Can you work these out from the model? Positions are in its coordinate system, mm. A direction names the side the tool comes from. Round coordinates to 2 decimals unless told otherwise and drop trailing zeros. Loops run counter-clockwise (first coordinate to the right, second up) from the corner with the lowest first, then second, coordinate; pieces in that order, holes last. Notation, with made-up numbers: (69, -26) -> (121, -26) arc R9 ccw to (121, -19) -> close; hole circle Ø7 at (53.5, 80). An arc over 180 degrees is marked (long way). Use a Markdown table: item, result.
from build123d import *

# Parameters (mm, degrees)
SKETCH1_W               = 26
SKETCH1_H               = 41
SKETCH1_R               = 1.375
SKETCH1_R_2             = 0.925
SKETCH1_H_2             = 4.4
BOSS_EXTRUDE1_DEPTH     = 6
SKETCH2_R               = 0.925
SKETCH2_R_2             = 1.375
BOSS_EXTRUDE2_DEPTH     = 15
CUT_EXTRUDE2_DEPTH      = 42.677451937
CUT_EXTRUDE2_DEPTH_BACK = 42.677451937
SKETCH4_W               = 26
SKETCH4_H               = 45.4
CUT_EXTRUDE1_DEPTH      = 7
FILLET1_R               = 2.2
FILLET2_R               = 2.2


with BuildPart() as part:
    # Sketch1 → Boss-Extrude1 (new body)
    # profile 1 of 2: a face of its own
    with BuildSketch(Plane(origin=(0, 0, 0), x_dir=(1, 0, 0), z_dir=(0, 1, 0))):
        Rectangle(SKETCH1_W, SKETCH1_H)
        with Locations(Location((-9, -18, 0), (0, 0, 270))):
            Circle(SKETCH1_R, mode=Mode.SUBTRACT)
        with BuildLine():
            ThreePointArc((10.375, -18), (9, -19.375), (7.625, -18))
            ThreePointArc((7.625, -18), (9, -16.625), (10.375, -18))
        make_face(mode=Mode.SUBTRACT)
        with Locations(Location((-9.5, 16, 0), (0, 0, 270))):
            Circle(SKETCH1_R_2, mode=Mode.SUBTRACT)
        with BuildLine():
            ThreePointArc((10.425, 16), (9.5, 15.075), (8.575, 16))
            ThreePointArc((8.575, 16), (9.5, 16.925), (10.425, 16))
        make_face(mode=Mode.SUBTRACT)
    # profile 2 of 2: a face of its own
    with BuildSketch(Plane(origin=(0, 0, 0), x_dir=(1, 0, 0), z_dir=(0, 1, 0))):
        with Locations((0, -22.7)):
            Rectangle(SKETCH1_W, SKETCH1_H_2)
    extrude(amount=BOSS_EXTRUDE1_DEPTH)

    # Sketch2 → Boss-Extrude2 (add)
    # profile 1 of 6: a face of its own
    with BuildSketch(Plane(origin=(0, 6, 0), x_dir=(1, 0, 0), z_dir=(0, 1, 0))):
        Polygon((12.587244228, 16.385905528), (10.85066935, 17.736574878), (9.114094472, 19.087244228), (0, 2.5), (4, 2.5), (4, 0), align=None)
        with BuildLine():
            ThreePointArc((10.425, 16), (8.669058384, 15.593599912), (10.067895068, 16.730150801))
            ThreePointArc((10.067895068, 16.730150801), (10.330941616, 16.406400088), (10.425, 16))
        make_face(mode=Mode.SUBTRACT)
    # profile 2 of 6: a face of its own
    with BuildSketch(Plane(origin=(0, 6, 0), x_dir=(1, 0, 0), z_dir=(0, 1, 0))):
        Polygon((-4, 0), (-4, 2.5), (0, 2.5), (-9.114094472, 19.087244228), (-12.587244228, 16.385905528), align=None)
        with Locations(Location((-9.5, 16, 0), (0, 0, 270))):
            Circle(SKETCH2_R, mode=Mode.SUBTRACT)
    # profile 3 of 6: a face of its own
    with BuildSketch(Plane(origin=(0, 6, 0), x_dir=(1, 0, 0), z_dir=(0, 1, 0))):
        Polygon((0, 2.5), (-4, 2.5), (-4, 0), (-4, -2.5), (0, -2.5), align=None)
    # profile 4 of 6: a face of its own
    with BuildSketch(Plane(origin=(0, 6, 0), x_dir=(1, 0, 0), z_dir=(0, 1, 0))):
        Polygon((4, 2.5), (0, 2.5), (0, -2.5), (4, -2.5), (4, 0), align=None)
    # profile 5 of 6: a face of its own
    with BuildSketch(Plane(origin=(0, 6, 0), x_dir=(1, 0, 0), z_dir=(0, 1, 0))):
        Polygon((12.482501962, -18.524099305), (4, 0), (4, -2.5), (0, -2.5), (7.724231954, -21.282516701), (10.103366958, -19.903308003), align=None)
        with BuildLine():
            ThreePointArc((10.375, -18), (10.191392249, -18.686447019), (9.689604349, -19.189567502))
            ThreePointArc((9.689604349, -19.189567502), (7.808607751, -17.313552981), (10.375, -18))
        make_face(mode=Mode.SUBTRACT)
    # profile 6 of 6: a face of its own
    with BuildSketch(Plane(origin=(0, 6, 0), x_dir=(1, 0, 0), z_dir=(0, 1, 0))):
        Polygon((-4, -2.5), (-4, 0), (-12.482501962, -18.524099305), (-7.724231954, -21.282516701), (0, -2.5), align=None)
        with Locations(Location((-9, -18, 0), (0, 0, 270))):
            Circle(SKETCH2_R_2, mode=Mode.SUBTRACT)
    extrude(amount=BOSS_EXTRUDE2_DEPTH)

    # Sketch6 → Cut-Extrude2 (cut, two sides: drawn at the far end of the back side and taken through both)
    with BuildSketch(Plane(origin=(13, 0, 0), x_dir=(0, 0, -1), z_dir=(1, 0, 0)).offset(-CUT_EXTRUDE2_DEPTH_BACK)):
        Polygon((-21.28, 17), (-21.28, 11), (-12.8, 11), (10.59, 17), align=None)
        Polygon((10.59, 12), (-12.8, 6), (19.09, 6), (19.09, 12), align=None)
        Polygon((-21.28, 21.511868699), (-21.28, 17), (10.59, 17), (19.087244228, 17), (19.087244228, 21.511868699), align=None)
    extrude(amount=CUT_EXTRUDE2_DEPTH + CUT_EXTRUDE2_DEPTH_BACK, mode=Mode.SUBTRACT)

    # Sketch4 → Cut-Extrude1 (cut)
    with BuildSketch(Plane.XZ):
        with Locations((0, 2.2)):
            Rectangle(SKETCH4_W, SKETCH4_H)
    extrude(amount=-CUT_EXTRUDE1_DEPTH, mode=Mode.SUBTRACT)

    # Fillet1
    # the kernel refuses this fillet: 2.2 mm, written as the material it takes off along each edge
    with BuildSketch(Plane(origin=(12.587244228, 7.402722975, -16.385905528), x_dir=(-0.46418305146339667, 0, 0.8857392927572592), z_dir=(0, 1, 0))) as fillet1_piece_1:
        with BuildLine():
            CenterArc((FILLET1_R * 0.83586855008, -FILLET1_R), FILLET1_R, 90, 79.782379698)
            Line((-FILLET1_R * 0.148272552074, -FILLET1_R * 0.822612596131), (0, 0))
            Line((0, 0), (FILLET1_R * 0.83586855008, 0))
        make_face()
    extrude(amount=14.194554051, mode=Mode.SUBTRACT)
    with BuildSketch(Plane(origin=(9.114094472, 5.550330565, -19.087244228), x_dir=(-0.48155808709989106, 0, 0.8764141764877459), z_dir=(0, 1, 0))) as fillet1_piece_2:
        with BuildLine():
            CenterArc((FILLET1_R * 1.17266716994, FILLET1_R), FILLET1_R, 170.912229019, 99.087770981)
            Line((FILLET1_R * 0.185219628956, FILLET1_R * 1.15794731336), (0, 0))
            Line((0, 0), (FILLET1_R * 1.17266716994, 0))
        make_face()
    extrude(amount=17.899338869, mode=Mode.SUBTRACT)
    with BuildSketch(Plane(origin=(-9.114094472, 5.550330565, -19.087244228), x_dir=(0.4815580870998917, 0, 0.8764141764877456), z_dir=(0, 1, 0))) as fillet1_piece_3:
        with BuildLine():
            CenterArc((FILLET1_R * 1.17266716994, -FILLET1_R), FILLET1_R, 90, 99.087770981)
            Line((FILLET1_R * 0.185219628956, -FILLET1_R * 1.15794731336), (0, 0))
            Line((0, 0), (FILLET1_R * 1.17266716994, 0))
        make_face()
    extrude(amount=17.899338869, mode=Mode.SUBTRACT)
    with BuildSketch(Plane(origin=(-12.587244228, 7.402722975, -16.385905528), x_dir=(0.46418305146339667, 0, 0.8857392927572592), z_dir=(0, 1, 0))) as fillet1_piece_4:
        with BuildLine():
            CenterArc((FILLET1_R * 0.83586855008, FILLET1_R), FILLET1_R, 190.217620302, 79.782379698)
            Line((-FILLET1_R * 0.148272552074, FILLET1_R * 0.822612596131), (0, 0))
            Line((0, 0), (FILLET1_R * 0.83586855008, 0))
        make_face()
    extrude(amount=14.194554051, mode=Mode.SUBTRACT)
    with BuildSketch(Plane(origin=(-12.482501962, 2.003928442, 18.524099305), x_dir=(0.4163419464168799, 0, -0.9092081080004752), z_dir=(0, 1, 0))) as fillet1_piece_5:
        with BuildLine():
            CenterArc((FILLET1_R * 0.908376646875, -FILLET1_R), FILLET1_R, 90, 84.502549141)
            Line((-FILLET1_R * 0.087023814771, -FILLET1_R * 0.904198533648), (0, 0))
            Line((0, 0), (FILLET1_R * 0.908376646875, 0))
        make_face()
    extrude(amount=13.992143116, mode=Mode.SUBTRACT)
    with BuildSketch(Plane(origin=(-7.724231954, 0.701160202, 21.282516701), x_dir=(0.3803394674675552, 0, -0.9248469546289788), z_dir=(0, 1, 0))) as fillet1_piece_6:
        with BuildLine():
            CenterArc((FILLET1_R * 1.14524359963, FILLET1_R), FILLET1_R, 172.25340707, 97.74659293)
            Line((FILLET1_R * 0.154369685137, FILLET1_R * 1.13479200861), (0, 0))
            Line((0, 0), (FILLET1_R * 1.14524359963, 0))
        make_face()
    extrude(amount=26.597679596, mode=Mode.SUBTRACT)
    with BuildSketch(Plane(origin=(12.482501962, 2.003928442, 18.524099305), x_dir=(-0.4163419464168806, 0, -0.9092081080004749), z_dir=(0, 1, 0))) as fillet1_piece_7:
        with BuildLine():
            CenterArc((FILLET1_R * 0.908376646875, FILLET1_R), FILLET1_R, 185.497450859, 84.502549141)
            Line((-FILLET1_R * 0.087023814771, FILLET1_R * 0.904198533648), (0, 0))
            Line((0, 0), (FILLET1_R * 0.908376646875, 0))
        make_face()
    extrude(amount=13.992143116, mode=Mode.SUBTRACT)
    with BuildSketch(Plane(origin=(7.724231954, 0.701160202, 21.282516701), x_dir=(-0.38033946746755576, 0, -0.9248469546289787), z_dir=(0, 1, 0))) as fillet1_piece_8:
        with BuildLine():
            CenterArc((FILLET1_R * 1.14524359963, -FILLET1_R), FILLET1_R, 90, 97.74659293)
            Line((FILLET1_R * 0.154369685137, -FILLET1_R * 1.13479200861), (0, 0))
            Line((0, 0), (FILLET1_R * 1.14524359963, 0))
        make_face()
    extrude(amount=26.597679596, mode=Mode.SUBTRACT)

    # Fillet2
    fillet2_edges = [part.edges().sort_by_distance(p)[0] for p in [
        (-4, 11.783454468, 0),
        (0, 12.424754168, -2.5),
        (4, 11.783454468, 0),
        (0, 11.142154767, 2.5),
    ]]
    fillet(fillet2_edges, radius=FILLET2_R)


solid = part.part
1. I need wall thicknesses on line 1 (X direction, y = 8.95, z = 18) (3 decimals); line 2 (X direction, y = 15.75, z = -15.5); line 3 (Y direction, x = 6.75, z = 17.5). Which ranges of each line are inside material? Lowest first, please.
Answer sheet:
| item | result |
|---|---|
| line 1 | x = -11.818 to -10.375, -7.625 to -6.374, 6.374 to 7.625, 10.375 to 11.818 |
| line 2 | x = -11.97 to -10.28, -8.72 to -7.14, 7.14 to 8.72, 10.28 to 11.97 |
| line 3 | y = 7 to 11 |
2. Will these pins go through, and if not, where does the flat tip stop? pin 1 Ø1.7 at (x, z) = (9, 18) entering from +Y; pin 2 Ø6 at (x, z) = (9.5, 16) entering from +Y; pin 3 Ø2 at (x, z) = (8, -15.5) entering from -Y; pin 4 Ø5 at (y, z) = (10, 6) entering from -X.
Answer sheet:
| item | result |
|---|---|
| pin 1 | passes through |
| pin 2 | stops at y = 11 |
| pin 3 | stops at y = 12 |
| pin 4 | stops at x = -7.89 |
3. I want a section at A-A (x = -5.25). Please give me the cut outline in (y, z).
Answer sheet:
| item | result |
|---|---|
| outline | (7, 8.9) -> (8.58, 2.73) -> (13.58, 2.73) -> (11, 12.8) -> (11, 15.27) -> (7, 15.27) -> close; (9.9, -2.39) -> (12, -10.59) -> (12, -12.05) -> (17, -12.05) -> (17, -10.59) -> (14.9, -2.39) -> close |
4. I want a section at D-D (x = 6). Please give me the cut outline in (y, z), plus the area to 3 significant figures.
Answer sheet:
| item | result |
|---|---|
| outline | (7, 8.9) -> (8.16, 4.37) -> (13.16, 4.37) -> (11, 12.8) -> (11, 17.09) -> (7, 17.09) -> close; (10.26, -3.82) -> (12, -10.59) -> (12, -13.42) -> (17, -13.42) -> (17, -10.59) -> (15.26, -3.82) -> close |
| area | 105 mm² |
5. If we mould it in two halves opening along Z, with no side actions, what happens to faces 1 (the cylindrical face through (-8.87, 14.46, -16.68)), 2 (the cylindrical face through (-8.1, 9, 20.2)), 3 (the flat face through (-8, 12, -14))? For each: +Z half, -Z half, draft (parallel to the pull), parting line (faces both ways), or undercut.
Answer sheet:
| item | result |
|---|---|
| face 1 | undercut |
| face 2 | +Z half |
| face 3 | draft |
6. Which directions (+Z, -Z, +X, -X, +Y, -Y) give clear straight access to the entire face, cutting with the end or side of a thin tool? Please do faces 4 (the flat face through (-8, 11, 16)), 5 (the flat face through (-8.168, 14.042, -7.953)), 6 (the flat face through (8.067, 14.042, -7.76)), 7 (the flat face through (4.94, 14.56, -11.49)).
Answer sheet:
| item | result |
|---|---|
| face 4 | +Z, +X, -X, +Y |
| face 5 | -X, +Y, -Y |
| face 6 | +X, +Y, -Y |
| face 7 | -Z, +Y, -Y |
7. I want a section at B-B (x = -9). Please give me the cut outline in (y, z) (3 decimals).
Answer sheet:
| item | result |
|---|---|
| outline | (7, 10.919) -> (11.483, 10.919) -> (11, 12.8) -> (11, 16.625) -> (7, 16.625) -> close; (7, 19.375) -> (11, 19.375) -> (11, 20.307) -> (7, 20.307) -> close; (11.731, -9.541) -> (12, -10.59) -> (12, -15.222) -> (17, -15.222) -> (17, -10.59) -> (16.731, -9.541) -> close; (12, -17.816) -> (17, -17.816) -> (17, -16.778) -> (12, -16.778) -> close |
8. I want a section at C-C (z = -3.5). Please give me the cut outline in (x, y), plus the area to 3 significant figures.
Answer sheet:
| item | result |
|---|---|
| outline | (-5.83, 10.18) -> (5.83, 10.18) -> (5.83, 15.18) -> (-5.83, 15.18) -> close |
| area | 58.3 mm² |
